Can you work these out from the drawing? Everything is in mm from the part's minimum corner. A direction names the side the tool comes from. Coordinates: 2 decimals unless noted, no trailing zeros. Loops run counter-clockwise (first coordinate to the right, second up) from the corner with the lowest first, then second, coordinate; pieces in that order, holes last. Notation, with made-up numbers: (-8, -4) -> (0, -4) arc R21 ccw to (0, 28) -> close; hole circle Ø10 at (17, -17). An arc over 180 degrees is marked (long way). One line per question, with ' | ' between items.
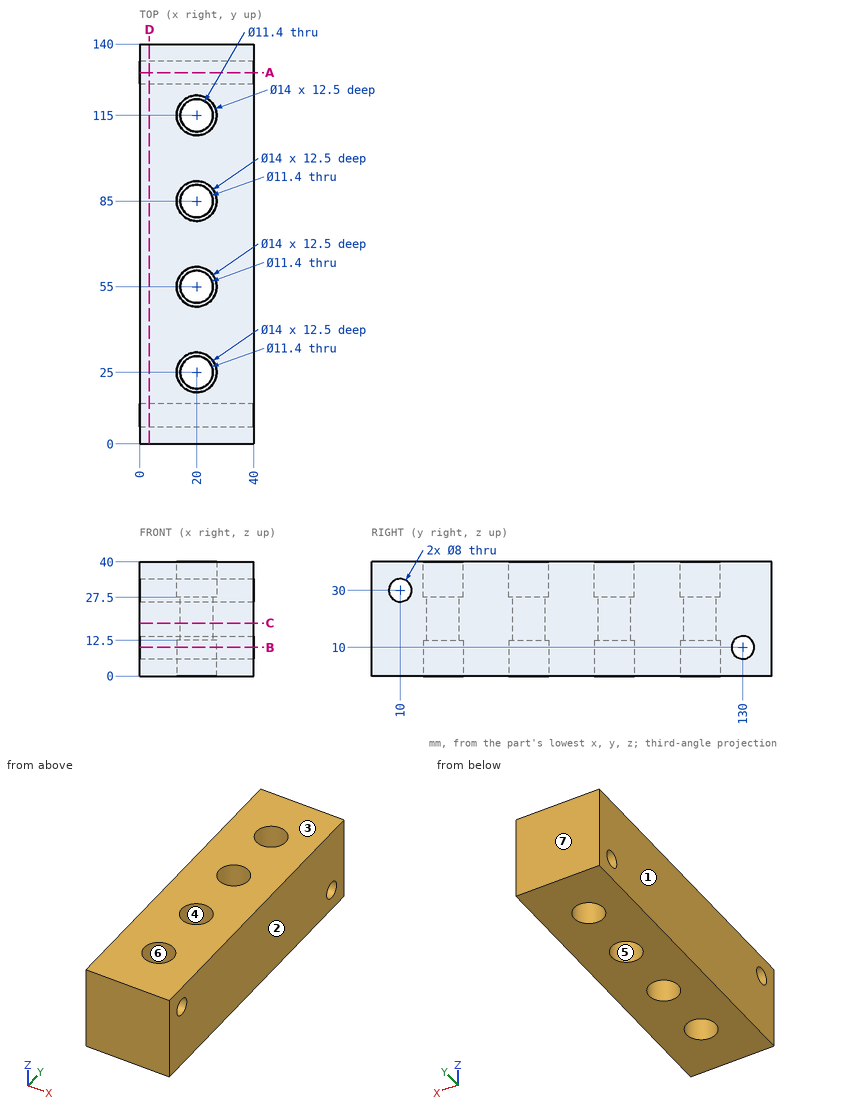
Q1. Imagine slicing it at D-D on x = 3.5. Write out the boundary of the cut face in (y, z), plus the area to 3 significant figures.
Values follow:
outline: (0, 0) -> (140, 0) -> (140, 40) -> (0, 40) -> close; hole circle Ø8 at (10, 30); hole circle Ø8 at (130, 10) | area: 5,500 mm2
Q2. Imagine slicing it at A-A on y = 130. Write out the boundary of the cut face in (x, z), plus the area to 3 significant figures.
Values follow:
outline: (0, 0) -> (40, 0) -> (40, 6) -> (0, 6) -> close; (0, 14) -> (40, 14) -> (40, 40) -> (0, 40) -> close | area: 1,280 mm2
Q3. Imagine slicing it at C-C on z = 18.5. Write out the boundary of the cut face in (x, y), plus the area to 3 significant figures.
Values follow:
outline: (0, 0) -> (40, 0) -> (40, 140) -> (0, 140) -> close; hole circle Ø11.4 at (20, 25); hole circle Ø11.4 at (20, 55); hole circle Ø11.4 at (20, 85); hole circle Ø11.4 at (20, 115) | area: 5,190 mm2
Q4. Please list where these lines run through material, in increasing order: L1, parallel to Y at x = 20, z = 37; L2, parallel to X at y = 55, z = 17; L3, parallel to Y at x = 20, z = 16. Write a range as [from, to].
Values follow:
L1: y = [0, 18], [32, 48], [62, 78], [92, 108], [122, 140] | L2: x = [0, 14.3], [25.7, 40] | L3: y = [0, 19.3], [30.7, 49.3], [60.7, 79.3], [90.7, 109.3], [120.7, 140]
Q5. For pin 1 (12.5 mm diameter, centred on x = 20, y = 85, fed in from -Z); pin 2 (7 mm diameter, centred on x = 22.5, y = 54, fed in from +Z), each with a flat end and sliding along its axis, tell me the tip position at first contact or that it passes through.
Values follow:
pin 1: stops at z = 12.5 | pin 2: stops at z = 27.5
Q6. We'd pull the mould along X, two halves only. Please class the marked faces 1, 2, 3 and 4: released by +X, released by -X, zero draft, split by the parting line, or undercut.
Values follow:
face 1: released by -X | face 2: released by +X | face 3: zero draft | face 4: undercut
Q7. Imagine slicing it at B-B on z = 10. Write out the boundary of the cut face in (x, y), plus the area to 3 significant figures.
Values follow:
outline: (0, 0) -> (40, 0) -> (40, 126) -> (0, 126) -> close; (0, 134) -> (40, 134) -> (40, 140) -> (0, 140) -> close; hole circle Ø14 at (20, 25); hole circle Ø14 at (20, 55); hole circle Ø14 at (20, 85); hole circle Ø14 at (20, 115) | area: 4,660 mm2
Q8. For the marked faces 5, 6 and 7, which set-ups out of +Z, -Z, +X, -X, +Y, -Y let a thin tool reach every point of the face, with its end or its side?
Values follow:
face 5: -Z | face 6: +Z | face 7: +Z, -Z, +X, -X, +Y
